Read the model definition and answer for the solid it produces. Units are mm, in the model's axes. A direction names the side the tool comes from. Round coordinates to 2 decimals unless told otherwise and drop trailing zeros. Write each loop counter-clockwise with the first axis right and the second up, starting at its lowest first coordinate (ties: lowest second). Pieces come first, ordered by that corner, then holes. Notation, with made-up numbers: (-22.5, -39) - (-1.5, -39) arc R32 ccw to (-1.5, -13) - close; hole circle Ø7 at (24, 22.5). An arc over 180 degrees is marked (long way). One line per item, written item: value. Start each with the question number.
(1) A cutting plane is placed at C-C, the plane z = 1.2. Determine the outline of the cut face in (x, y), plus the area to 3 significant figures.
(2) A cutting plane is placed at D-D, the plane y = -5. Determine the outline of the cut face in (x, z).
(3) A cutting plane is placed at A-A, the plane y = 0. Determine the outline of the cut face in (x, z), plus the area to 3 significant figures.
(4) For faces 1 (the face through (-5.7, -5, 1)), 2 (the face through (8, -3.5, 1)), 3 (the face through (0, -2, 2)), determine the directions among +Z, -Z, +X, -X, +Y, -Y from which every point of the face is accessible in a straight line to the end or side of a thin tool.
(5) Flat-ended cylindrical pins translate along their axes: pin 1 Ø1 at (y, z) = (-6, 1) entering from +X; pin 2 Ø1 at (y, z) = (4, 0.5) entering from +X. Find the tip coordinate at first contact, or state that the pin passes through.
(6) Find the intervals of material crossed by L1, parallel to Y at x = 0, z = 0.8; L2, parallel to X at y = -0.75, z = 1.7; L3, parallel to X at y = -5, z = 0.25, in increasing order.
(7) The mould has two halves that part along Y. Classify faces 4 (the face through (9.7, -2, 1)), 5 (the face through (7.989, 4.696, 0.986)), 6 (the face through (-1.5, 0.07, 0.99)): +Y half, -Y half, draft (parallel to the pull), parting line (faces both ways), or undercut.
(8) A cutting plane is placed at B-B, the plane x = 0. Determine the outline of the cut face in (y, z), plus the area to 3 significant figures.
from build123d import *

# Parameters (mm, degrees)
MODEL_R             = 1.5
BOSS_EXTRUDE1_DEPTH = 2


with BuildPart() as part:
    # Model → Boss-Extrude1 (new body)
    with BuildSketch(Plane.XY):
        with BuildLine():
            Line((9.7, -3.5), (9.7, 0.5))
            ThreePointArc((9.7, 0.5), (7.942640687, 4.742640687), (3.7, 6.5))
            Line((3.7, 6.5), (-3.7, 6.5))
            ThreePointArc((-3.7, 6.5), (-7.942640687, 4.742640687), (-9.7, 0.5))
            Line((-9.7, 0.5), (-9.7, -3.5))
            Line((-9.7, -3.5), (-5.7, -3.5))
            Line((-5.7, -3.5), (-5.7, -7.5))
            Line((-5.7, -7.5), (5.7, -7.5))
            Line((5.7, -7.5), (5.7, -3.5))
            Line((5.7, -3.5), (9.7, -3.5))
        make_face()
        Circle(MODEL_R, mode=Mode.SUBTRACT)
    extrude(amount=BOSS_EXTRUDE1_DEPTH)


solid = part.part
Here are the results:
1. outline: (-9.7, -3.5) - (-5.7, -3.5) - (-5.7, -7.5) - (5.7, -7.5) - (5.7, -3.5) - (9.7, -3.5) - (9.7, 0.5) arc R6 ccw to (3.7, 6.5) - (-3.7, 6.5) arc R6 ccw to (-9.7, 0.5) - close; hole circle Ø3 at (0, 0)
1. area: 217 mm²
2. outline: (-5.7, 0) - (5.7, 0) - (5.7, 2) - (-5.7, 2) - close
3. outline: (-9.7, 0) - (-1.5, 0) - (-1.5, 2) - (-9.7, 2) - close; (1.5, 0) - (9.7, 0) - (9.7, 2) - (1.5, 2) - close
3. area: 32.8 mm²
4. face 1: +Z, -Z, -X, -Y
4. face 2: +Z, -Z, +X, -Y
4. face 3: +Z, +X, -X, +Y, -Y
5. pin 1: x = 5.7
5. pin 2: x = 8.9
6. L1: -7.5 to -1.5, 1.5 to 6.5
6. L2: -9.7 to -1.3, 1.3 to 9.7
6. L3: -5.7 to 5.7
7. face 4: draft
7. face 5: +Y half
7. face 6: undercut
8. outline: (-7.5, 0) - (-1.5, 0) - (-1.5, 2) - (-7.5, 2) - close; (1.5, 0) - (6.5, 0) - (6.5, 2) - (1.5, 2) - close
8. area: 22.0 mm²
